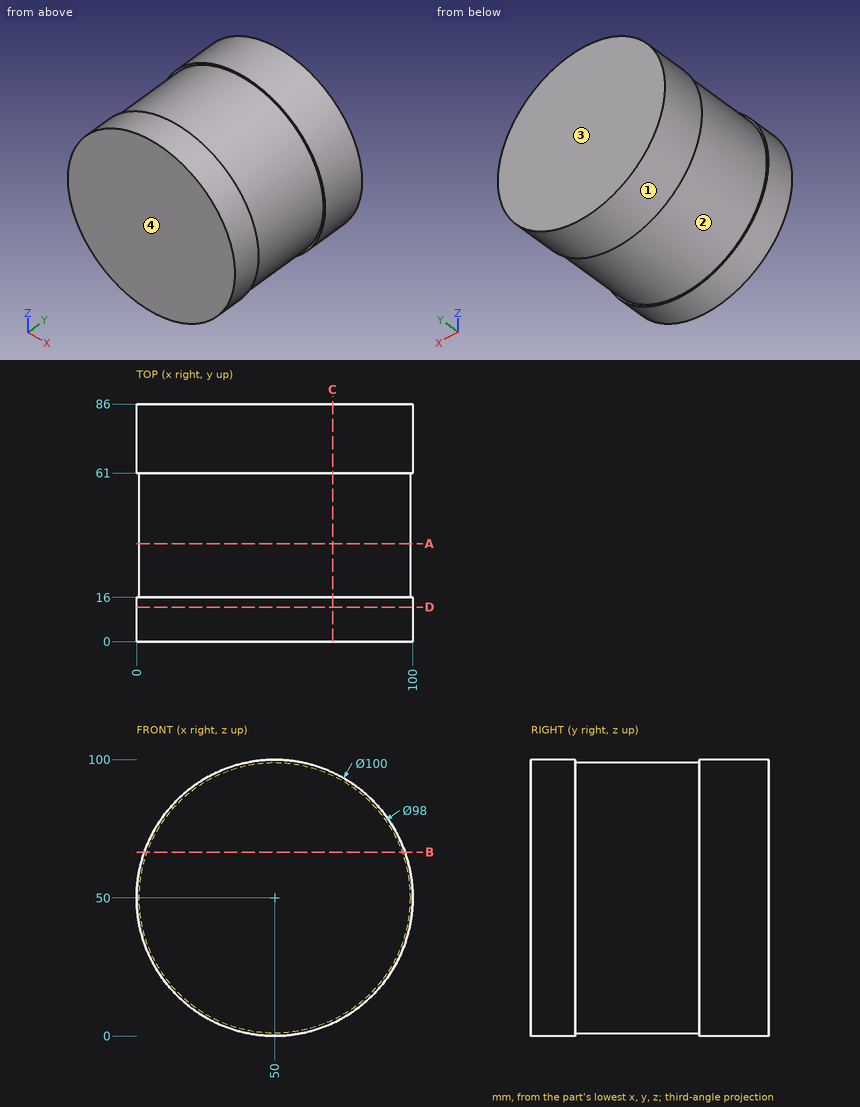
Drawing for the job (mm, zero at the part's lowest x, y, z). Round coordinates to 2 decimals unless told otherwise and drop trailing zeros. Loops run counter-clockwise (first coordinate to the right, second up) from the corner with the lowest first, then second, coordinate; pieces in that order, holes last. Notation, with made-up numbers: (19, 59) -> (38, 59) arc R18 ccw to (38, 93) -> close; hole circle Ø1 at (32, 30.25). An arc over 180 degrees is marked (long way). Use one line per item in the form item = value. Start each with the question number.
Item 1: Band-saw the part on C-C (x = 71). List the corners of the cut face in (y, z).
Item 2: Drop flat-ended pins along their axis: pin 1 Ø2 at (x, y) = (72, 39) entering from -Z; pin 2 Ø10 at (y, z) = (12.5, 43) entering from -X; pin 3 Ø1 at (y, z) = (46, 40) entering from -X. Give the stop position or say it passes through.
Item 3: Band-saw the part on A-A (y = 35.5). List the corners of the cut face in (x, z).
Item 4: Two-plate mould, pull along Y, no slides. Class the marked faces 1, 2, 3 and 4: released by +Y, released by -Y, zero draft, split by the parting line, or undercut.
Item 5: Drill centre lines: line 1 along X through (y, z) = (46, 50); line 2 along X through (y, z) = (81.5, 32); line 3 along Z through (x, y) = (52, 55). Where is each one in solid material? Low to high.
Item 6: Band-saw the part on D-D (y = 12.5). List the corners of the cut face in (x, z).
Item 7: Band-saw the part on B-B (z = 66.5). List the corners of the cut face in (x, y).
Data:
q1.outline = (0, 4.62) -> (16, 4.62) -> (16, 5.73) -> (61, 5.73) -> (61, 4.62) -> (86, 4.62) -> (86, 95.38) -> (61, 95.38) -> (61, 94.27) -> (16, 94.27) -> (16, 95.38) -> (0, 95.38) -> close
q2.pin_1 = 5.73
q2.pin_2 = 0.04
q2.pin_3 = 1.93
q3.outline = circle Ø98 at (50, 50)
q4.face_1 = zero draft
q4.face_2 = undercut
q4.face_3 = released by +Y
q4.face_4 = released by -Y
q5.line_1 = 1 to 99
q5.line_2 = 3.35 to 96.65
q5.line_3 = 1.04 to 98.96
q6.outline = circle Ø100 at (50, 50)
q7.outline = (2.8, 0) -> (97.2, 0) -> (97.2, 16) -> (96.14, 16) -> (96.14, 61) -> (97.2, 61) -> (97.2, 86) -> (2.8, 86) -> (2.8, 61) -> (3.86, 61) -> (3.86, 16) -> (2.8, 16) -> close
